Geometry: see drawing. Coordinates: mm, zero at the bounding-box minimum. A direction names the side the tool comes from. Coordinates: 2 decimals unless noted, no trailing zeros. Write each loop counter-clockwise with the first axis right and the second up, starting at its lowest first coordinate (ties: lowest second). Pieces come first, ordered by that corner, then holes. Notation, with made-up numbers: M -5.5,87.5 L 27.5,87.5 A27 ccw 27.5,123.5 Z; hole C -23.75,79.5 d1. An arc over 180 degrees is marked long. Answer as CSV lines item,"result". Start each with the question number.
1. Section D-D on y = 17.5. Return the cut outline in (x, z), plus the area to 3 significant figures.
2. Line query: probe 1 along Y at (x, z) = (17.5, 3.25); probe 2 along X at (y, z) = (17.5, 3.25). Output: solid intervals per line, ascending. Write a range as [from, to].
3. Section C-C on z = 7.5. Return the cut outline in (x, y), plus the area to 3 significant figures.
4. Mould query, pull axis Y, two halves, no side actions, for the marked faces 4, 5 and 6. Classes: pulls with the +Y half, pulls with the -Y half, needs draft (parallel to the pull), parting line crosses it, or undercut.
5. Reachability of the marked faces 1, 2 and 3 from +Z, -Z, +X, -X, +Y, -Y: full face, straight path, thin tool, end or side. Return the list, or none.
6. Section A-A on x = 17.5. Return the cut outline in (y, z), plus the area to 3 significant figures.
7. Contact query for flat-ended pins moving along their axis: pin 1 Ø12 at (x, y) = (17, 58.5) entering from +Z; pin 2 Ø1.5 at (y, z) = (58.5, 11.5) entering from -X; pin 3 Ø10.5 at (x, y) = (19, 17) entering from -Z; pin 4 Ø8 at (x, z) = (26, 10) entering from +Y. Output: stop coordinate, or through.
8. Section B-B on z = 3.75. Return the cut outline in (x, y).
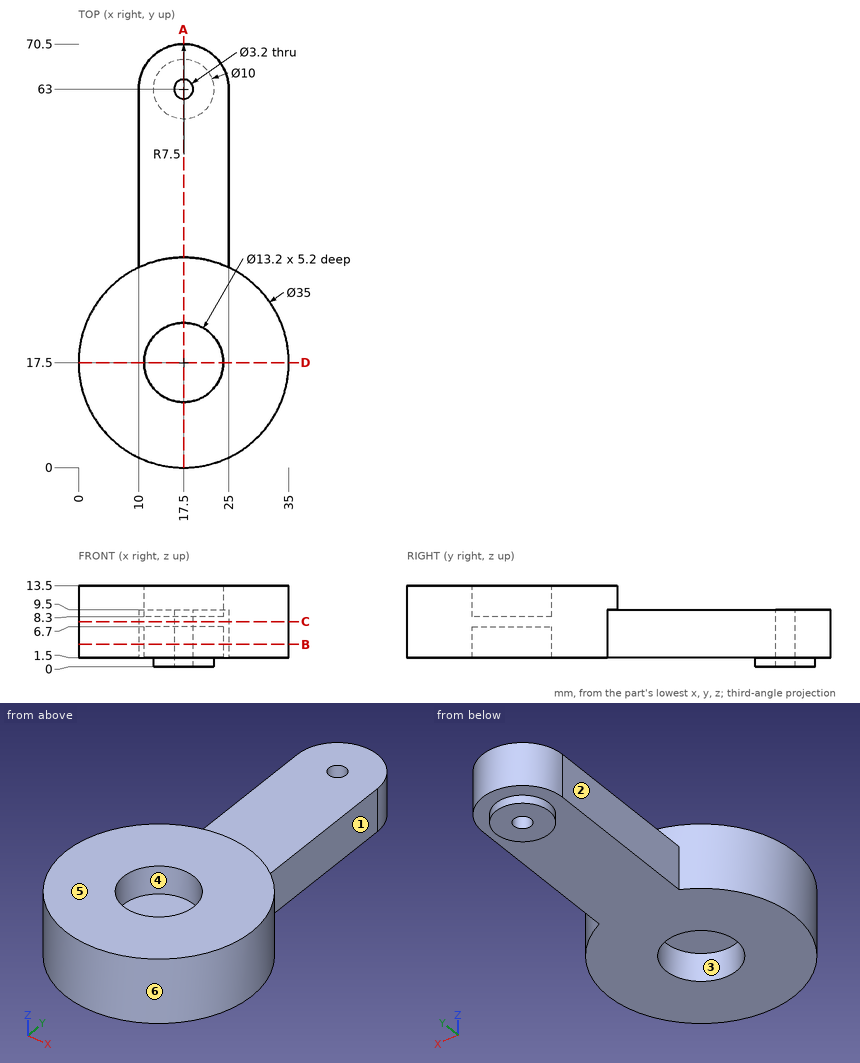
Values:
1,outline,"M 0,1.5 L 10.9,1.5 L 10.9,6.7 L 24.1,6.7 L 24.1,1.5 L 35,1.5 L 35,13.5 L 24.1,13.5 L 24.1,8.3 L 10.9,8.3 L 10.9,13.5 L 0,13.5 Z"
1,area,"283 mm²"
2,probe 1,"[0, 10.9], [24.1, 61.4], [64.6, 70.5]"
2,probe 2,"[0, 10.9], [24.1, 35]"
3,outline,"M 10,33.31 A17.5 ccw long 25,33.31 L 25,63 A7.5 ccw 10,63 Z; hole C 17.5,63 d3.2"
3,area,"1,470 mm²"
4,face 4,"undercut"
4,face 5,"needs draft"
4,face 6,"parting line crosses it"
5,face 1,"+Z, -Z, +X, +Y"
5,face 2,"+Z, -Z, -X, +Y"
5,face 3,"-Z"
6,outline,"M 0,1.5 L 10.9,1.5 L 10.9,6.7 L 24.1,6.7 L 24.1,1.5 L 58,1.5 L 58,0 L 61.4,0 L 61.4,9.5 L 35,9.5 L 35,13.5 L 24.1,13.5 L 24.1,8.3 L 10.9,8.3 L 10.9,13.5 L 0,13.5 Z; M 64.6,0 L 68,0 L 68,1.5 L 70.5,1.5 L 70.5,9.5 L 64.6,9.5 Z"
6,area,"551 mm²"
7,pin 1,"z = 9.5"
7,pin 2,"through"
7,pin 3,"z = 1.5"
7,pin 4,"y = 68.98"
8,outline,"M 10,33.31 A17.5 ccw long 25,33.31 L 25,63 A7.5 ccw 10,63 Z; hole C 17.5,17.5 d13.2; hole C 17.5,63 d3.2"
